from build123d import *

# Parameters (mm, degrees)
SKETCH1_W           = 175
SKETCH1_H           = 92
BOSS_EXTRUDE1_DEPTH = 24
SKETCH2_W           = 171
SKETCH2_H           = 85
CUT_EXTRUDE1_DEPTH  = 22
SKETCH3_W           = 25
SKETCH3_H           = 12
CUT_EXTRUDE2_DEPTH  = 2
SKETCH4_W           = 5
SKETCH4_H           = 3.5
CUT_EXTRUDE4_DEPTH  = 2
SKETCH5_W           = 5
SKETCH5_H           = 3.5
CUT_EXTRUDE7_DEPTH  = 2
SKETCH7_W           = 2
SKETCH7_H           = 5
CUT_EXTRUDE8_DEPTH  = 2
SKETCH10_W          = 2
SKETCH10_H          = 5
CUT_EXTRUDE9_DEPTH  = 2
SKETCH11_W          = 2
SKETCH11_H          = 5
CUT_EXTRUDE10_DEPTH = 2


with BuildPart() as part:
    # Sketch1 → Boss-Extrude1 (new body)
    with BuildSketch(Plane(origin=(0, 0, 0), x_dir=(1, 0, 0), z_dir=(0, 1, 0))):
        Rectangle(SKETCH1_W, SKETCH1_H)
    extrude(amount=BOSS_EXTRUDE1_DEPTH)

    # Sketch2 → Cut-Extrude1 (cut)
    with BuildSketch(Plane(origin=(0, 24, 0), x_dir=(1, 0, 0), z_dir=(0, 1, 0))):
        Rectangle(SKETCH2_W, SKETCH2_H)
    extrude(amount=-CUT_EXTRUDE1_DEPTH, mode=Mode.SUBTRACT)

    # Sketch3 → Cut-Extrude2 (cut)
    with BuildSketch(Plane.ZY.offset(87.5)):
        with Locations((0, 18)):
            Rectangle(SKETCH3_W, SKETCH3_H)
    extrude(amount=-CUT_EXTRUDE2_DEPTH, mode=Mode.SUBTRACT)

    # Sketch4 → Cut-Extrude4 (cut)
    with BuildSketch(Plane(origin=(0, 24, 0), x_dir=(1, 0, 0), z_dir=(0, 1, 0))):
        with Locations((-80, 44.25)):
            Rectangle(SKETCH4_W, SKETCH4_H)
        with Locations((-40, 44.25)):
            Rectangle(SKETCH4_W, SKETCH4_H)
        with Locations((0, 44.25)):
            Rectangle(SKETCH4_W, SKETCH4_H)
        with Locations((40, 44.25)):
            Rectangle(SKETCH4_W, SKETCH4_H)
        with Locations((80, 44.25)):
            Rectangle(SKETCH4_W, SKETCH4_H)
    extrude(amount=-CUT_EXTRUDE4_DEPTH, mode=Mode.SUBTRACT)

    # Sketch5 → Cut-Extrude7 (cut)
    with BuildSketch(Plane(origin=(0, 24, 0), x_dir=(1, 0, 0), z_dir=(0, 1, 0))):
        with Locations((-80, -44.25)):
            Rectangle(SKETCH5_W, SKETCH5_H)
        with Locations((-40, -44.25)):
            Rectangle(SKETCH5_W, SKETCH5_H)
        with Locations((0, -44.25)):
            Rectangle(SKETCH5_W, SKETCH5_H)
        with Locations((40, -44.25)):
            Rectangle(SKETCH5_W, SKETCH5_H)
        with Locations((80, -44.25)):
            Rectangle(SKETCH5_W, SKETCH5_H)
    extrude(amount=-CUT_EXTRUDE7_DEPTH, mode=Mode.SUBTRACT)

    # Sketch7 → Cut-Extrude8 (cut)
    with BuildSketch(Plane(origin=(0, 24, 0), x_dir=(1, 0, 0), z_dir=(0, 1, 0))):
        with Locations((86.5, 0)):
            Rectangle(SKETCH7_W, SKETCH7_H)
        with Locations((86.5, -34)):
            Rectangle(SKETCH7_W, SKETCH7_H)
        with Locations((86.5, 34)):
            Rectangle(SKETCH7_W, SKETCH7_H)
    extrude(amount=-CUT_EXTRUDE8_DEPTH, mode=Mode.SUBTRACT)

    # Sketch10 → Cut-Extrude9 (cut)
    with BuildSketch(Plane(origin=(0, 24, 0), x_dir=(1, 0, 0), z_dir=(0, 1, 0))):
        with Locations((-86.5, 34)):
            Rectangle(SKETCH10_W, SKETCH10_H)
    extrude(amount=-CUT_EXTRUDE9_DEPTH, mode=Mode.SUBTRACT)

    # Sketch11 → Cut-Extrude10 (cut)
    with BuildSketch(Plane(origin=(0, 24, 0), x_dir=(1, 0, 0), z_dir=(0, 1, 0))):
        with Locations((-86.5, -34)):
            Rectangle(SKETCH11_W, SKETCH11_H)
    extrude(amount=-CUT_EXTRUDE10_DEPTH, mode=Mode.SUBTRACT)


solid = part.part
Geometry check sheet. Reference: the model listing, model coordinates, mm. A direction names the side the tool comes from. Give positions to 0.01 mm unless a question says otherwise; leave off trailing zeros. Order: outer loops, then holes, each group sorted by start corner. A loop starts at its lowest first (then second) coordinate and runs counter-clockwise, first axis right, second up. Notation, with made-up numbers: (78, 37.5) - (106, 37.5) arc R22 ccw to (106, 70.5) - close; hole circle Ø9 at (19, 47.25). An arc over 180 degrees is marked (long way). Use one line per item in the form item = value.
1) Sectioned sample at C-C (z = 9.5). Record the boundary of the cut face in (x, y), and give its area (3 significant figures).
Working result:
outline = (-87.5, 0) - (87.5, 0) - (87.5, 24) - (85.5, 24) - (85.5, 2) - (-85.5, 2) - (-85.5, 12) - (-87.5, 12) - close
area = 414 mm^2
2) Sectioned sample at B-B (y = 18). Record the boundary of the cut face in (x, z), and give its area (4 significant figures).
Working result:
outline = (-87.5, -46) - (87.5, -46) - (87.5, 46) - (-87.5, 46) - (-87.5, 12.5) - (-85.5, 12.5) - (-85.5, 42.5) - (85.5, 42.5) - (85.5, -42.5) - (-85.5, -42.5) - (-85.5, -12.5) - (-87.5, -12.5) - close
area = 1,515 mm^2
3) Access from +Z, -Z, +X, -X, +Y, -Y to the whole of each face (thin tool, end or side, straight path). Record for faces 3 (the face through (-1, 13, 42.5)), 4 (the face through (60, 24, -44)), 5 (the face through (80, 22, 44)).
Working result:
face_3 = +Y
face_4 = +Z, -Z, +X, -X, +Y
face_5 = +Z, -Z, +Y
4) Material ranges on probe 1 along X at (y, z) = (2.5, 32.5); probe 2 along Z at (x, y) = (-43.5, 23); probe 3 along Y at (x, z) = (-53.5, -38), recorded low to high. Write a range as from..to.
Working result:
probe_1 = -87.5..-85.5, 85.5..87.5
probe_2 = -46..-42.5, 42.5..46
probe_3 = 0..2
5) Draft check along X on faces 1 (the face through (-1, 0, -1)), 2 (the face through (-1, 2, -1)). Enter one of: released by +X, released by -X, zero draft, split by the parting line, or undercut.
Working result:
face_1 = zero draft
face_2 = undercut
6) Sectioned sample at A-A (y = 6.5). Record the boundary of the cut face in (x, z), and give its area (4 significant figures).
Working result:
outline = (-87.5, -46) - (87.5, -46) - (87.5, 46) - (-87.5, 46) - close; hole (-85.5, -42.5) - (85.5, -42.5) - (85.5, 42.5) - (-85.5, 42.5) - close
area = 1,565 mm^2
7) Sectioned sample at D-D (x = 8). Record the boundary of the cut face in (y, z).
Working result:
outline = (0, -46) - (24, -46) - (24, -42.5) - (2, -42.5) - (2, 42.5) - (24, 42.5) - (24, 46) - (0, 46) - close
8) Depth check by flat-ended pin: pin 1 Ø1.8 at (x, z) = (-40, -44) entering from +Y; pin 2 Ø1 at (x, z) = (-86, 2.5) entering from +Y; pin 3 Ø8 at (x, z) = (-11.5, -0.5) entering from +Y. Enter the tip coordinate at first touch or a pass-through.
Working result:
pin_1 = 22
pin_2 = 12
pin_3 = 2
